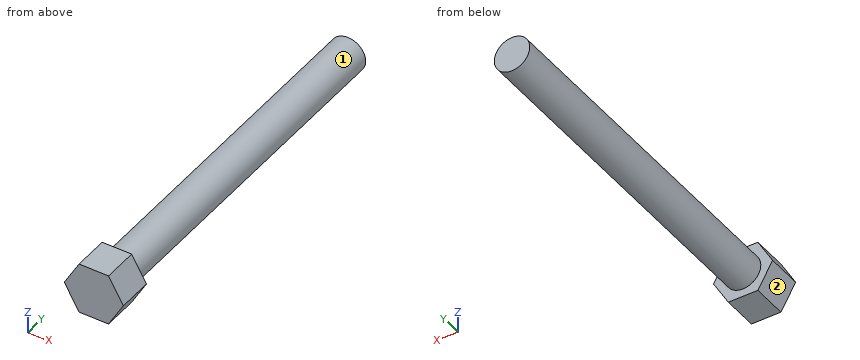
from build123d import *

# Parameters (mm, degrees)
SKETCH1_R           = 1.5
BOSS_EXTRUDE1_DEPTH = 30
BOSS_EXTRUDE2_DEPTH = 3


with BuildPart() as part:
    # Sketch1 → Boss-Extrude1 (new body)
    with BuildSketch(Plane(origin=(0, 0, 0), x_dir=(1, 0, 0), z_dir=(0, 1, 0))):
        with Locations(Location((0, 0, 0), (0, 0, 270))):
            Circle(SKETCH1_R)
    extrude(amount=BOSS_EXTRUDE1_DEPTH)

    # Sketch2 → Boss-Extrude2 (add)
    with BuildSketch(Plane.XZ):
        Polygon((1.25, -2.165063509), (2.5, 0), (1.25, 2.165063509), (-1.25, 2.165063509), (-2.5, 0), (-1.25, -2.165063509), align=None)
    extrude(amount=BOSS_EXTRUDE2_DEPTH)


solid = part.part
Can you work these out from the model? Positions are in its coordinate system, mm. Face numbers are marked on the shaded views. A direction names the side the tool comes from. Give positions to 0.01 mm unless a question says otherwise; leave off trailing zeros. Loops run counter-clockwise (first coordinate to the right, second up) from the corner with the lowest first, then second, coordinate; pieces in that order, holes last. Notation, with made-up numbers: (27, 82.25) - (40, 82.25) arc R28 cw to (40, 110.25) - close; hole circle Ø10 at (82, -36.5). An arc over 180 degrees is marked (long way). Answer as a JSON object with one key per item and string values.
Q1. Imagine slicing it at D-D on x = 1.8. Write out the boundary of the cut face in (y, z), plus the area to 3 significant figures.
Geometry says:
{"outline": "(-3, -1.21) - (0, -1.21) - (0, 1.21) - (-3, 1.21) - close", "area": "7.27 mm²"}
Q2. Which directions (+Z, -Z, +X, -X, +Y, -Y) give clear straight access to the entire face, cutting with the end or side of a thin tool? Please do the marked faces 1 and 2.
Geometry says:
{"face 1": "+Y", "face 2": "-Z, -X, +Y, -Y"}
Q3. If I drill on L1, parallel to X at y = 23.5, z = 0.1; L2, parallel to Y at x = -1.7, z = 0.9; L3, parallel to X at y = 29, z = -1.2, over which ranges is the centre line in solid material (lowest first)?
Geometry says:
{"L1": "-1.5 to 1.5", "L2": "-3 to 0", "L3": "-0.9 to 0.9"}
Q4. Imagine slicing it at C-C on x = -2. Write out the boundary of the cut face in (y, z), plus the area to 3 significant figures.
Geometry says:
{"outline": "(-3, -0.87) - (0, -0.87) - (0, 0.87) - (-3, 0.87) - close", "area": "5.20 mm²"}
Q5. Imagine slicing it at B-B on y = 26.5. Write out the boundary of the cut face in (x, z).
Geometry says:
{"outline": "circle Ø3 at (0, 0)"}
Q6. Imagine slicing it at A-A on x = 0. Write out the boundary of the cut face in (y, z), plus the area to 3 significant figures.
Geometry says:
{"outline": "(-3, -2.17) - (0, -2.17) - (0, -1.5) - (30, -1.5) - (30, 1.5) - (0, 1.5) - (0, 2.17) - (-3, 2.17) - close", "area": "103 mm²"}
